Geometry check sheet. Reference: the model listing, model coordinates, mm. A direction names the side the tool comes from. Give positions to 0.01 mm unless a question says otherwise; leave off trailing zeros. Loops run counter-clockwise (first coordinate to the right, second up) from the corner with the lowest first, then second, coordinate; pieces in that order, holes last. Notation, with made-up numbers: (-22.5, 58.5) -> (-2.5, 58.5) arc R29 ccw to (-2.5, 89.5) -> close; hole circle Ø7 at (0.5, -23). An arc over 180 degrees is marked (long way). Write item = value, one per line.
```python
from build123d import *

# Parameters (mm, degrees)
BOSS_EXTRUDE1_DEPTH = 841.375
SKETCH2_R           = 12.7
CUT_EXTRUDE1_DEPTH  = 3.175
LPATTERN1_COUNT     = 4
LPATTERN1_PITCH     = 420.6875


with BuildPart() as part:
    # Sketch1 → Boss-Extrude1 (new body, symmetric)
    with BuildSketch(Plane(origin=(0, 0, 0), x_dir=(0, 0, -1), z_dir=(1, 0, 0))):
        with BuildLine():
            Line((33.3248, 25.4), (-33.3248, 25.4))
            ThreePointArc((-33.3248, 25.4), (-36.701376302, 24.001376302), (-38.1, 20.6248))
            Line((-38.1, 20.6248), (-38.1, 4.7752))
            ThreePointArc((-38.1, 4.7752), (-36.701376302, 1.398623698), (-33.3248, 0))
            Line((-33.3248, 0), (33.3248, 0))
            ThreePointArc((33.3248, 0), (36.701376302, 1.398623698), (38.1, 4.7752))
            Line((38.1, 4.7752), (38.1, 20.6248))
            ThreePointArc((38.1, 20.6248), (36.701376302, 24.001376302), (33.3248, 25.4))
        make_face()
        with BuildLine():
            Line((33.3248, 22.225), (-33.3248, 22.225))
            ThreePointArc((-33.3248, 22.225), (-34.456312271, 21.756312271), (-34.925, 20.6248))
            Line((-34.925, 20.6248), (-34.925, 4.7752))
            ThreePointArc((-34.925, 4.7752), (-34.456312271, 3.643687729), (-33.3248, 3.175))
            Line((-33.3248, 3.175), (33.3248, 3.175))
            ThreePointArc((33.3248, 3.175), (34.456312271, 3.643687729), (34.925, 4.7752))
            Line((34.925, 4.7752), (34.925, 20.6248))
            ThreePointArc((34.925, 20.6248), (34.456312271, 21.756312271), (33.3248, 22.225))
        make_face(mode=Mode.SUBTRACT)
    extrude(amount=BOSS_EXTRUDE1_DEPTH, both=True)

    # Sketch2 → Cut-Extrude1 (cut)
    with BuildSketch(Plane(origin=(0, 25.4, 0), x_dir=(1, 0, 0), z_dir=(0, 1, 0))):
        with Locations((-631.03125, 0)):
            Circle(SKETCH2_R)
    cut_extrude1 = extrude(amount=-CUT_EXTRUDE1_DEPTH, mode=Mode.SUBTRACT)

    # LPattern1: Cut-Extrude1 ×4
    with Locations(*[(i * LPATTERN1_PITCH, 0, 0) for i in range(1, LPATTERN1_COUNT)]):
        add(cut_extrude1, mode=Mode.SUBTRACT)


solid = part.part
```
Item 1: Tool access check on faces 1 (the flat face through (12, 22.225, 0)), 2 (the flat face through (12, 0, 0)), 3 (the cylindrical face through (618.344, 23.835, -0.558)). Record the directions out of +Z, -Z, +X, -X, +Y, -Y that give a thin tool (end or side, any length) a straight path to the whole face; none if there is none.
Answer:
face_1 = +X, -X
face_2 = +Z, -Z, +X, -X, -Y
face_3 = +Y
Item 2: Section check A-A, the plane y = 16. Record the cut outline in (x, z) (3 decimals), plus the area to 3 significant figures.
Answer:
outline = (-841.375, -38.1) -> (841.375, -38.1) -> (841.375, -34.925) -> (-841.375, -34.925) -> close; (-841.375, 34.925) -> (841.375, 34.925) -> (841.375, 38.1) -> (-841.375, 38.1) -> close
area = 10,700 mm^2
Item 3: Section check C-C, the plane z = 0. Record the cut outline in (x, y) (3 decimals), plus the area to 3 significant figures.
Answer:
outline = (-841.375, 0) -> (841.375, 0) -> (841.375, 3.175) -> (-841.375, 3.175) -> close; (-841.375, 22.225) -> (-643.731, 22.225) -> (-643.731, 25.4) -> (-841.375, 25.4) -> close; (-618.331, 22.225) -> (-223.044, 22.225) -> (-223.044, 25.4) -> (-618.331, 25.4) -> close; (-197.644, 22.225) -> (197.644, 22.225) -> (197.644, 25.4) -> (-197.644, 25.4) -> close; (223.044, 22.225) -> (618.331, 22.225) -> (618.331, 25.4) -> (223.044, 25.4) -> close; (643.731, 22.225) -> (841.375, 22.225) -> (841.375, 25.4) -> (643.731, 25.4) -> close
area = 10,400 mm^2
Item 4: Section check B-B, the plane x = 509. Record the cut outline in (y, z) (3 decimals), plus the area to 3 significant figures.
Answer:
outline = (0, -33.325) arc R4.775 ccw to (4.775, -38.1) -> (20.625, -38.1) arc R4.775 ccw to (25.4, -33.325) -> (25.4, 33.325) arc R4.775 ccw to (20.625, 38.1) -> (4.775, 38.1) arc R4.775 ccw to (0, 33.325) -> close; hole (3.175, -33.325) arc R1.6 ccw to (4.775, -34.925) -> (20.625, -34.925) arc R1.6 ccw to (22.225, -33.325) -> (22.225, 33.325) arc R1.6 ccw to (20.625, 34.925) -> (4.775, 34.925) arc R1.6 ccw to (3.175, 33.325) -> close
area = 587 mm^2
Item 5: Draft check along Z on faces 4 (the flat face through (12, 25.4, 0)), 5 (the cylindrical face through (-643.72, 23.83, -0.56)), 6 (the cylindrical face through (222.075, 23.835, 4.864)). Enter one of: +Z half, -Z half, draft (parallel to the pull), parting line (faces both ways), or undercut.
Answer:
face_4 = draft
face_5 = undercut
face_6 = undercut
Item 6: Thickness scan on L1, parallel to X at y = 24.4, z = 0 (3 decimals); L2, parallel to Z at x = -127, y = 19 (3 decimals); L3, parallel to Y at x = -736.5, z = -0.5 (3 decimals). Record the ranges inside material, lowest first. Write a range as [from, to].
Answer:
L1 = [-841.375, -643.731], [-618.331, -223.044], [-197.644, 197.644], [223.044, 618.331], [643.731, 841.375]
L2 = [-38.1, -34.925], [34.925, 38.1]
L3 = [0, 3.175], [22.225, 25.4]
Item 7: Gauge pin test, flat ends, axial feed: pin 1 (3 mm diameter, centred on x = 461, y = 22.5, fed in from -Z); pin 2 (23 mm diameter, centred on x = 210.34, z = 0, fed in from +Y) (3 decimals); pin 3 (4 mm diameter, centred on y = 20, z = 22, fed in from +X). Record the tip position at first contact, or that the pin passes through.
Answer:
pin_1 = -38.09
pin_2 = 3.175
pin_3 = through
